Build history of the part. All positions in model axes, mm. Face numbers are marked on the shaded views. A direction names the side the tool comes from. Give positions to 0.01 mm unless a question says otherwise; leave off trailing zeros. Write each loop counter-clockwise with the first axis right and the second up, starting at its lowest first coordinate (ties: lowest second). Pieces come first, ordered by that corner, then holes. Notation, with made-up numbers: (-21.5, -6.75) -> (-8.5, -6.75) arc R26 ccw to (-8.5, 27.25) -> close; hole circle Ø4 at (21.25, -7.5). An arc over 180 degrees is marked (long way). One line per question, with ' | ' between items. Start each with the question number.
(1) Band-saw the part on A-A, the plane z = 0. Give the cut face in (x, y) (3 decimals).
(2) Band-saw the part on B-B, the plane y = 14.5. Give the cut face in (x, z) (3 decimals), and give its area (3 significant figures).
(3) Pin check, flat tips, straight feed: P1, Ø2, axis at x = -31.5, y = 4, coming from the -Z side; P2, Ø9, axis at x = -26, z = 23, coming from the +Y side; P3, Ø4, axis at y = 15, z = 3.5, coming from the -X side. Stop position of each tip, or through.
(4) Tool access for the marked faces 4, 5 and 6: list every direction of +Z, -Z, +X, -X, +Y, -Y with a clear straight run to the whole face (end or side of a thin tool).
(5) Pull direction Z, two halves, no side cores. Call the marked faces 1, 2 and 3: released by +Z, released by -Z, zero draft, split by the parting line, or undercut.
(6) Drill centre lines: probe 1 along X at (y, z) = (30, 11); probe 2 along X at (y, z) = (27, -11); probe 3 along Z at (x, y) = (-11, 29). Where is each one in solid material? Low to high. Write a range as from..to.
from build123d import *

# Parameters (mm, degrees)
CBORE_FOR_M4_SHCS1_D           = 4.5
CBORE_FOR_M4_SHCS1_CBORE_D     = 8
CBORE_FOR_M4_SHCS1_CBORE_DEPTH = 4
M3X0_5_TAPPED_HOLE1_D          = 2.5
M8X1_0_TAPPED_HOLE1_D          = 7
M8X1_0_TAPPED_HOLE1_DEPTH      = 21
M8X1_0_TAPPED_HOLE1_TIP        = 2.103012167
HOLE1_D                        = 4.4
HOLE1_CBORE_D                  = 7.85
HOLE1_CBORE_DEPTH              = 1.27
CUT_EXTRUDE1_DEPTH             = 1
CUT_EXTRUDE1_DEPTH_BACK        = 33
CUT_EXTRUDE2_REACH             = 79.279
M3X0_5_TAPPED_HOLE2_D          = 2.5
M3X0_5_TAPPED_HOLE2_DEPTH      = 7.5
M3X0_5_TAPPED_HOLE2_TIP        = 0.751075774


with BuildPart() as part:
    # Sketch1 → Revolve1 (revolve)
    with BuildSketch(Plane.XY):
        Polygon((10.235, 32), (10.235, 25), (25, 25), (29.55, 10), (29.55, 0), (40, 0), (40, 28.1), (21.75, 28.1), (20.25, 32), align=None)
    revolve(axis=Axis((0, 10.573566085, 0), (0, -1, 0)))

    # CBORE for M4 SHCS1 (through all)
    with Locations(Plane(origin=(0, 28.1, 0), x_dir=(1, 0, 0), z_dir=(0, 1, 0))):
        with Locations((-24.04163056, 24.04163056), (24.04163056, 24.04163056), (24.04163056, -24.04163056), (-24.04163056, -24.04163056)):
            CounterBoreHole(CBORE_FOR_M4_SHCS1_D / 2, CBORE_FOR_M4_SHCS1_CBORE_D / 2, CBORE_FOR_M4_SHCS1_CBORE_DEPTH)

    # M3x0.5 Tapped Hole1 (through all)
    with Locations(Plane(origin=(0, 32, 0), x_dir=(1, 0, 0), z_dir=(0, 1, 0))):
        with Locations((-11, 11), (11, 11), (11, -11), (-11, -11), (0, 15.556349186), (15.556349186, 0), (0, -15.556349186), (-15.556349186, 0)):
            Hole(M3X0_5_TAPPED_HOLE1_D / 2)

    # M8x1.0 Tapped Hole1
    with Locations(Plane(origin=(0, 28.1, 0), x_dir=(1, 0, 0), z_dir=(0, 1, 0))):
        with Locations((31.508719031, 12.775), (31.508719031, -12.775)):
            Hole(M8X1_0_TAPPED_HOLE1_D / 2, depth=M8X1_0_TAPPED_HOLE1_DEPTH)
            with Locations((0, 0, -(M8X1_0_TAPPED_HOLE1_DEPTH + M8X1_0_TAPPED_HOLE1_TIP / 2))):  # 118° drill point
                Cone(0, M8X1_0_TAPPED_HOLE1_D / 2, M8X1_0_TAPPED_HOLE1_TIP, mode=Mode.SUBTRACT)

    # Hole1 (through all)
    with Locations(Plane(origin=(0, 0, 0), x_dir=(-1, 0, 0), z_dir=(0, -1, 0))):
        with Locations((-31.508719031, -12.775), (-31.508719031, 12.775)):
            CounterBoreHole(HOLE1_D / 2, HOLE1_CBORE_D / 2, HOLE1_CBORE_DEPTH)

    # Sketch13 → Cut-Extrude1 (cut, two sides)
    with BuildSketch(Plane.XZ) as cut_extrude1_sk:
        with BuildLine():
            Line((-37.279350853, 14.5), (-37.279350853, -14.5))
            ThreePointArc((-37.279350853, -14.5), (-40, 0), (-37.279350853, 14.5))
        make_face()
    extrude(amount=CUT_EXTRUDE1_DEPTH, mode=Mode.SUBTRACT)
    extrude(cut_extrude1_sk.sketch, amount=-CUT_EXTRUDE1_DEPTH_BACK, mode=Mode.SUBTRACT)

    # Sketch14 → Cut-Extrude2 (cut, up to next)
    with BuildSketch(Plane.ZY.offset(37.279350853), mode=Mode.PRIVATE) as cut_extrude2_sk1:
        with BuildLine():
            Line((-7, 7.358571571), (-7, 0))
            Line((-7, 0), (7, 0))
            Line((7, 0), (7, 7.358571571))
            ThreePointArc((7, 7.358571571), (0, 24.5), (-7, 7.358571571))
        make_face()
    cut_extrude2_tool1 = extrude(cut_extrude2_sk1.sketch, amount=-CUT_EXTRUDE2_REACH, mode=Mode.PRIVATE) & part.part
    add(cut_extrude2_tool1.solids().sort_by_distance((-37.279351, 12.225831, 0))[0], mode=Mode.SUBTRACT)

    # M3x0.5 Tapped Hole2
    with Locations(Plane.ZY.offset(37.279350853)):
        with Locations((-11, 25.5), (-11, 3.5), (11, 3.5), (11, 25.5)):
            Hole(M3X0_5_TAPPED_HOLE2_D / 2, depth=M3X0_5_TAPPED_HOLE2_DEPTH)
            with Locations((0, 0, -(M3X0_5_TAPPED_HOLE2_DEPTH + M3X0_5_TAPPED_HOLE2_TIP / 2))):  # 118° drill point
                Cone(0, M3X0_5_TAPPED_HOLE2_D / 2, M3X0_5_TAPPED_HOLE2_TIP, mode=Mode.SUBTRACT)


solid = part.part
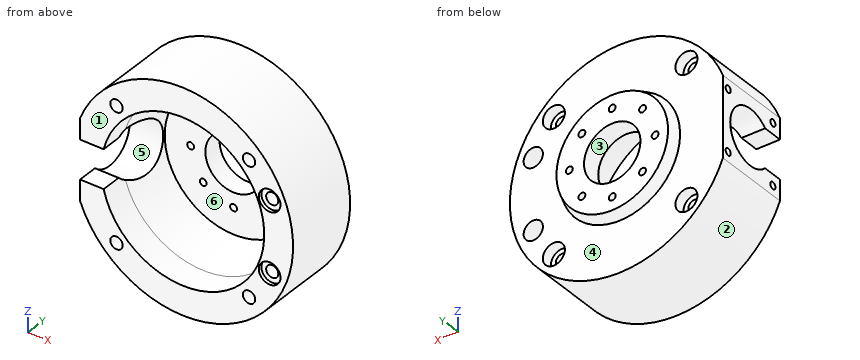
Results:
1) outline: (-37.279, 24.5) -> (-25.152, 24.5) -> (-25, 25) -> (-16.806, 25) -> (-16.806, 32) -> (-20.25, 32) -> (-21.75, 28.1) -> (-37.279, 28.1) -> close; (-14.306, 25) -> (-10.235, 25) -> (-10.235, 32) -> (-14.306, 32) -> close; (10.235, 25) -> (14.306, 25) -> (14.306, 32) -> (10.235, 32) -> close; (16.806, 25) -> (25, 25) -> (29.55, 10) -> (29.55, 0) -> (40, 0) -> (40, 28.1) -> (21.75, 28.1) -> (20.25, 32) -> (16.806, 32) -> close
2) outline: (-37.279, -14.5) arc R40 ccw (long way) to (-37.279, 14.5) -> (-37.279, 10) -> (-26.351, 10) arc R28.185 cw (long way) to (-26.351, -10) -> (-37.279, -10) -> close; hole circle Ø4.5 at (-24.042, -24.042); hole circle Ø4.5 at (-24.042, 24.042); hole circle Ø4.5 at (24.042, -24.042); hole circle Ø4.5 at (24.042, 24.042); hole circle Ø7 at (31.509, -12.775); hole circle Ø7 at (31.509, 12.775) | area: 2,140 mm²
3) P1: stops at z = -25.88 | P2: stops at y = 28.1 | P3: stops at x = 27.14
4) face 4: +Y | face 5: -X | face 6: -Y
5) face 1: zero draft | face 2: split by the parting line | face 3: undercut
6) probe 1: x = -17.91..-12.25, -9.75..9.75, 12.25..17.91 | probe 2: x = -37.28..-12.25, -9.75..9.75, 12.25..28.49, 34.53..38.46 | probe 3: z = -18.36..-12.25, -9.75..9.75, 12.25..18.36
